from build123d import *

# Parameters (mm, degrees)
SKETCH001_R = 2
SKETCH002_R = 1.5
SKETCH003_R = 1.5
SKETCH004_R = 0.5
SKETCH_R    = 3.25


with BuildPart() as loft001:
    # Sketch001 → Loft001 section 0
    with BuildSketch(Plane.XY.offset(2.5)):
        Circle(SKETCH001_R)
    # Sketch002 → Loft001 section 1
    with BuildSketch(Plane.XY.offset(4)):
        Circle(SKETCH002_R)
    loft()


with BuildPart() as loft002:
    # Sketch002 → Loft002 section 0
    with BuildSketch(Plane.XY.offset(4)):
        Circle(SKETCH002_R)
    # Sketch003 → Loft002 section 1
    with BuildSketch(Plane.XY.offset(27)):
        Circle(SKETCH003_R)
    loft()


with BuildPart() as loft003:
    # Sketch003 → Loft003 section 0
    with BuildSketch(Plane.XY.offset(27)):
        Circle(SKETCH003_R)
    # Sketch004 → Loft003 section 1
    with BuildSketch(Plane.XY.offset(30)):
        Circle(SKETCH004_R)
    loft()


with BuildPart() as fusion:
    # Sketch → Loft section 0
    with BuildSketch(Plane.XY):
        Circle(SKETCH_R)
    # Sketch001 → Loft section 1
    with BuildSketch(Plane.XY.offset(2.5)):
        Circle(SKETCH001_R)
    loft()

    # Fusion: union Loft001, Loft002, Loft003
    add(loft001.part)
    add(loft002.part)
    add(loft003.part)


solid = fusion.part
Source: CAD feature listing. Evaluate the final solid. Frame: model axes, mm. A direction names the side the tool comes from. Give positions to 0.01 mm unless a question says otherwise; leave off trailing zeros. Order: outer loops, then holes, each group sorted by start corner. A loop starts at its lowest first (then second) coordinate and runs counter-clockwise, first axis right, second up. Notation, with made-up numbers: (25.25, 20) -> (83.25, 20) arc R30 ccw to (83.25, 54) -> close; hole circle Ø1 at (-35, -21). An arc over 180 degrees is marked (long way). Write item = value, one per line.
Q1. Cut plane A-A, the plane x = 0. Output: boundary loops of the cut face in (y, z).
Data:
outline = (-3.25, 0) -> (3.25, 0) -> (2, 2.5) -> (1.5, 4) -> (1.5, 27) -> (0.5, 30) -> (-0.5, 30) -> (-1.5, 27) -> (-1.5, 4) -> (-2, 2.5) -> close
Q2. Pin query (flat end, axial travel): pin 1 (1 mm diameter, centred on x = 1.5, z = 21, fed in from +Y); pin 2 (1.5 mm diameter, centred on x = 0.5, z = 19, fed in from +Y); pin 3 (3 mm diameter, centred on x = 1, y = 1.5, fed in from +Z); pin 4 (3 mm diameter, centred on y = -1, z = 26.5, fed in from +X). Return the tip coordinate at first contact, or that it passes through.
Data:
pin_1 = 1.12
pin_2 = 1.5
pin_3 = 30
pin_4 = 1.5
Q3. Cut plane B-B, the plane z = 24.5. Output: boundary loops of the cut face in (x, y).
Data:
outline = circle Ø3 at (0, 0)
Q4. Material intervals for line 1 (Z direction, x = -2, y = 1.5); line 2 (X direction, y = -0.5, z = 20.5); line 3 (Y direction, x = -1, z = 21.5), sorted ascending. Write a range as from..to.
Data:
line_1 = 0..1.5
line_2 = -1.41..1.41
line_3 = -1.12..1.12
Q5. Set-up query: faces 1 (the face through (-1.5, 0.07, 15.66)), 2 (the face through (0, 0, 30)). Return all of +Z, -Z, +X, -X, +Y, -Y with unobstructed straight access to the full face (end or side cutting, diameter ignored); none if empty.
Data:
face_1 = +Z
face_2 = +Z, +X, -X, +Y, -Y
